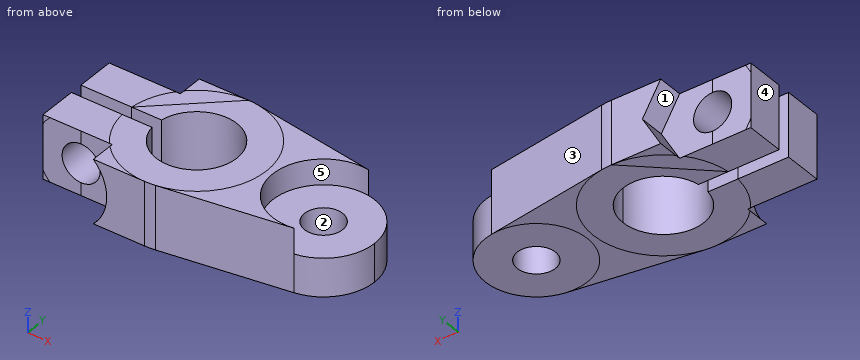
Autodesk Inventor part; units mm, degrees
ref_plane "YZ Plane" through (0, 0, 0) normal (1, 0, 0) x (0, 1, 0)
ref_plane "XZ Plane" through (0, 0, 0) normal (0, 1, 0) x (-1, 0, 0)
ref_plane "XY Plane" through (0, 0, 0) normal (0, 0, 1) x (1, 0, 0)
sketch "Sketch1" plane through (0, 0, 0) normal (0, 0, 1) x (1, 0, 0)
  circle A0 centre (0, 0) radius 3.175
  circle A1 centre (0, 0) radius 5.5
  circle A2 centre (10, 0) radius 4
  line L0 (0.825, 5.4378) -> (10.6, 3.9547)
  line L1 (0.825, -5.4378) -> (10.6, -3.9547)
  circle A3 centre (10, 0) radius 1.5
  dimension "d0" = 6.35
  dimension "d1" = 11
  dimension "d2" = 8
  dimension "d3" = 10
  dimension "d4" = 3
extrude "Extrusion1" add sketch "Sketch1" along normal blind 5
sketch "Sketch2" plane through (0, 0, 5) normal (0, 0, 1) x (1, 0, 0)
  arc A0 (0.825, 5.4378) -> (0.825, -5.4378) centre (0, 0) ccw
  line L0 (0, -5.5) -> (-9.4772, -5.5)
  line L1 (-9.4772, -5.5) -> (-9.4772, -0.5)
  line L2 (-9.4772, -0.5) -> (-5.4772, -0.5)
  line L3 (-5.4772, -0.5) -> (0, -5.5)
  line L4 (0, 5.5) -> (-9.4772, 5.5)
  line L5 (-9.4772, 5.5) -> (-9.4772, 0.5)
  line L6 (-9.4772, 0.5) -> (-5.4772, 0.5)
  line L7 (-5.4772, 0.5) -> (0, 5.5)
  line L8 (-7.4772, -0.5) -> (-7.4772, 0.5) construction
  point P0 (-7.4772, 0)
  dimension "d7" = 1
  dimension "d8" = 4
extrude "Extrusion2" add sketch "Sketch2" against normal blind 5 contours L7 A0 | A0 L6 L5 L4 | A0 L0 L1 L2
sketch "Sketch3" plane through (-9.4772, -5.5, 5) normal (0, -1, 0) x (1, 0, 0)
  line L0 (0, 0) -> (4, 0) construction
  line L1 (0, 0) -> (0, -5) construction
  line L2 (4, -5) -> (0, -5) construction
  line L3 (4, 0) -> (4, -5) construction
  line L4 (0, 0) -> (4, 0) construction
  line L5 (2, 0) -> (2, -5) construction
  circle A0 centre (3, -2.5) radius 1.5
  point P0 (9.4772, -5)
  point P1 (2, -2.5)
  dimension "d11" = 3
  dimension "d12" = 1
extrude "Extrusion3" cut sketch "Sketch3" against normal through all
sketch "Sketch4" plane through (0, 0, 5) normal (0, 0, 1) x (1, 0, 0)
  line L0 (-9.4772, 0.5) -> (0, 0.5)
  line L1 (0, 0.5) -> (0, -0.5)
  line L2 (0, -0.5) -> (-9.4772, -0.5)
  line L3 (-9.4772, -0.5) -> (-9.4772, 0.5)
  point P0 (0, 0)
  point P1 (0, 0)
extrude "Extrusion4" cut sketch "Sketch4" against normal through all
sketch "Sketch5" plane through (-9.4772, 5.5, 5) normal (0, 1, 0) x (1, 0, 0)
  circle A0 centre (3, 2.5) radius 1.5
  line L0 (7.0415, 2.5) -> (5.0207, -1)
  line L1 (5.0207, -1) -> (0.9793, -1)
  line L2 (0.9793, -1) -> (-1.0415, 2.5)
  line L3 (-1.0415, 2.5) -> (0.9793, 6)
  line L4 (0.9793, 6) -> (5.0207, 6)
  line L5 (5.0207, 6) -> (7.0415, 2.5)
  point P0 (9.4772, 5)
  dimension "d17" = 7
extrude "Extrusion5" cut sketch "Sketch5" against normal blind 2 contours A0 | L0 L1 L2 L3 L4 L5
sketch "Sketch6" plane through (-9.4772, -5.5, 5) normal (0, -1, 0) x (1, 0, 0)
  circle A0 centre (3, -2.5) radius 1.5
  circle A1 centre (3, -2.5) radius 3.5
  point P0 (9.4772, -5)
  dimension "d20" = 7
extrude "Extrusion6" cut sketch "Sketch6" against normal blind 2 contours A0 | A1
sketch "Sketch7" plane through (0, 0, 5) normal (0, 0, 1) x (1, 0, 0)
  circle A0 centre (10, 0) radius 1.5
  arc A1 (10.6, -3.9547) -> (10.6, 3.9547) centre (10, 0) ccw
  circle A2 centre (10, 0) radius 4
  point P0 (0, 0)
extrude "Extrusion7" cut sketch "Sketch7" against normal blind 2
sketch "Sketch8" plane through (-9.4772, -3.5, 5) normal (0, -1, 0) x (1, 0, 0)
  line L0 (5.4495, -5) -> (0.5505, -5)
  line L1 (0, 0) -> (0, -5)
  line L2 (3, -5) -> (0, -5)
  line L3 (0, -5) -> (0, 0)
  line L4 (0, 0) -> (3, 0)
  line L5 (3, 0) -> (3, -5)
  point P0 (9.4772, -5)
extrude "Extrusion8" cut sketch "Sketch8" along normal through all
sketch "Sketch9" plane through (-9.4772, 3.5, 5) normal (0, 1, 0) x (1, 0, 0)
  circle A0 centre (3, 2.5) radius 1.5
  line L0 (5.5981, 0) -> (0.4019, 0)
  line L1 (0, 0) -> (0, 5)
  line L2 (3, 0) -> (0, 0)
  line L3 (0, 0) -> (0, 5)
  line L4 (0, 5) -> (3, 5)
  line L5 (3, 5) -> (3, 0)
  point P0 (9.4772, 5)
extrude "Extrusion9" cut sketch "Sketch9" along normal through all contours L5 A0 | A0 L5 L0 L2 L1 L4 picked at (2.8803, 2.0145)
properties part number "TA08" material "ABS Plastic"
Could you check a few things on this model? Use its own coordinates, in mm. Face numbers are marked on the shaded views. A direction names the side the tool comes from. Give positions to 0.01 mm unless a question says otherwise; leave off trailing zeros. Loops run counter-clockwise (first coordinate to the right, second up) from the corner with the lowest first, then second, coordinate; pieces in that order, holes last. Notation, with made-up numbers: M 20.25,78.5 L 74.25,78.5 A29 ccw 74.25,110.5 Z; hole C 25,24.5 d10. An arc over 180 degrees is marked long. Answer as a JSON object with one key per item and string values.
Q1. For P1, Ø3, axis at x = -7, z = 2, coming from the -Y side; P2, Ø2.5, axis at x = -6.48, z = 2.5, coming from the -Y side; P3, Ø1.2, axis at x = -5.5, z = 2.5, coming from the +Y side, each with a flat end and sliding along its axis, tell me the tip position at first contact or that it passes through.
Values found:
{"P1": "stops at y = -3.5", "P2": "passes through", "P3": "stops at y = 3.5"}
Q2. For the marked faces 4 and 5, which set-ups out of +Z, -Z, +X, -X, +Y, -Y let a thin tool reach every point of the face, with its end or its side?
Values found:
{"face 4": "+Z, -Z, -X, +Y, -Y", "face 5": "+Z"}
Q3. Suppose I cut it at A-A, the plane y = -0.75. List the corners of the cut face in (x, z) for me, plus the area to 3 significant figures.
Values found:
{"outline": "M -9.48,0 L -3.09,0 L -3.09,5 L -9.48,5 Z; M 3.09,0 L 8.7,0 L 8.7,3 L 6.07,3 L 6.07,5 L 3.09,5 Z; M 11.3,0 L 13.93,0 L 13.93,3 L 11.3,3 Z; hole C -6.48,2.5 d3", "area": "55.6 mm²"}
Q4. If I drill on probe 1 along X at (y, z) = (1.25, 3.1); probe 2 along X at (y, z) = (1.2, 2.5); probe 3 along Y at (x, z) = (-7.75, 3.75), over which ranges is the centre line in solid material (lowest first)? Write a range as [from, to].
Values found:
{"probe 1": "x = [-9.48, -7.85], [-5.1, -2.92], [2.92, 6.2]", "probe 2": "x = [-9.48, -7.98], [-4.98, -2.94], [2.94, 9.1], [10.9, 13.82]", "probe 3": "y = [-3.5, -0.5], [0.5, 3.5]"}
Q5. Suppose I cut it at B-B, the plane x = 1.75. List the corners of the cut face in (y, z) for me.
Values found:
{"outline": "M -5.3,0 L -2.65,0 L -2.65,5 L -5.3,5 Z; M 2.65,0 L 5.3,0 L 5.3,5 L 2.65,5 Z"}
Q6. Suppose I cut it at D-D, the plane y = 2.25. List the corners of the cut face in (x, z) for me, plus the area to 3 significant figures.
Values found:
{"outline": "M -9.48,0 L -2.24,0 L -2.24,5 L -9.48,5 Z; M 2.24,0 L 13.31,0 L 13.31,3 L 6.69,3 L 6.69,5 L 2.24,5 Z; hole C -6.48,2.5 d3", "area": "71.2 mm²"}
Q7. Suppose I cut it at C-C, the plane z = 2. List the corners of the cut face in (x, y) for me (3 decimals), plus the area to 3 significant figures.
Values found:
{"outline": "M -9.477,-3.5 L -7.891,-3.5 L -7.891,-0.5 L -9.477,-0.5 Z; M -9.477,0.5 L -7.891,0.5 L -7.891,3.5 L -9.477,3.5 Z; M -5.063,-3.5 L -3.013,-3.5 L -3.013,-5.5 L 0,-5.5 A5.5 ccw 0.825,-5.438 L 10.6,-3.955 A4 ccw 10.6,3.955 L 0.825,5.438 A5.5 ccw 0,5.5 L -2.724,5.5 L -2.724,3.5 L -5.063,3.5 L -5.063,0.5 L -3.135,0.5 A3.175 cw long -3.135,-0.5 L -5.063,-0.5 Z; hole C 10,0 d3", "area": "137 mm²"}
Q8. If we mould it in two halves opening along X, with no side actions, what happens to the marked faces 1, 2 and 3? For each: pulls with the +X half, pulls with the -X half, needs draft (parallel to the pull), parting line crosses it, or undercut.
Values found:
{"face 1": "pulls with the -X half", "face 2": "undercut", "face 3": "pulls with the +X half"}
